```python
from build123d import *

# Parameters (mm, degrees)
BASE_FLANGE1_DEPTH = 20.1168
SKETCH6_R          = 2.4892
CUT_EXTRUDE1_DEPTH = 72.471393622
SKETCH7_R          = 5.08
CUT_EXTRUDE2_DEPTH = 71.156041481
FILLET1_R          = 3.175


# Read off the part's stored shape, not the designer's step: Base-Flange1
with BuildPart() as part:
    # Base-Flange1 outline → Base-Flange1 (new body)
    with BuildSketch(Plane(origin=(0, 0, 0), x_dir=(1, 0, 0), z_dir=(0, 1, 0))):
        with BuildLine():
            Line((3.429, 0), (63.5, 0))
            Line((63.5, 0), (63.5, 2.667))
            Line((63.5, 2.667), (3.429, 2.667))
            ThreePointArc((3.429, 2.667), (2.890184633, 2.890184633), (2.667, 3.429))
            Line((2.667, 3.429), (2.667, 28.575))
            Line((2.667, 28.575), (0, 28.575))
            Line((0, 28.575), (0, 3.429))
            ThreePointArc((0, 3.429), (1.004330847, 1.004330847), (3.429, 0))
        make_face()
    extrude(amount=BASE_FLANGE1_DEPTH)

    # Sketch6 → Cut-Extrude1 (cut, through all)
    with BuildSketch(Plane(origin=(0, 0, -2.667), x_dir=(-1, 0, 0), z_dir=(0, 0, -1))):
        with Locations((-50.8, 10.0584)):
            Circle(SKETCH6_R)
        with Locations((-38.1, 10.0584)):
            Circle(SKETCH6_R)
        with Locations((-25.4, 10.0584)):
            Circle(SKETCH6_R)
        with Locations((-12.7, 10.0584)):
            Circle(SKETCH6_R)
    extrude(amount=-CUT_EXTRUDE1_DEPTH, mode=Mode.SUBTRACT)

    # Sketch7 → Cut-Extrude2 (cut, through all)
    with BuildSketch(Plane(origin=(2.667, 0, 0), x_dir=(0, 0, -1), z_dir=(1, 0, 0))):
        with Locations((19.05, 10.0584)):
            Circle(SKETCH7_R)
    extrude(amount=-CUT_EXTRUDE2_DEPTH, mode=Mode.SUBTRACT)

    # Fillet1
    fillet1_edges = [part.edges().sort_by_distance(p)[0] for p in [
        (1.3335, 20.1168, -28.575),
        (1.3335, 0, -28.575),
        (63.5, 20.1168, -1.3335),
        (63.5, 0, -1.3335),
    ]]
    fillet(fillet1_edges, radius=FILLET1_R)


solid = part.part
```
For this review, take the finished solid that the model builds, in its own axes (mm). A direction names the side the tool comes from. Give positions to 0.01 mm unless a question says otherwise; leave off trailing zeros. Write each loop counter-clockwise with the first axis right and the second up, starting at its lowest first coordinate (ties: lowest second). Pieces come first, ordered by that corner, then holes.
Item 1: Wall thickness on probe 1 along Y at (x, z) = (38.1, -1.6); probe 2 along X at (y, z) = (13.75, -26); probe 3 along Z at (x, y) = (61.5, 18): over which ranges is each line inside the solid? List them lowest first.
Item 2: Take a section at A-A (y = 14.25). Give the boundary of the cut face in (x, z) (3 decimals), and give its area (3 significant figures).
Item 3: Machinability: for faces 5 (the face through (62.545, 19.211, -1.352)), 6 (the face through (34, 10, -2.667)), which of the approach directions +Z, -Z, +X, -X, +Y, -Y give a long, thin tool a straight path to every point of the face, cutting with its end or side? Answer none if there is none.
Item 4: Take a section at B-B (x = 25.4). Give the boundary of the cut face in (y, z).
Item 5: Take a section at C-C (z = -19.05). Give the boundary of the cut face in (x, y).
Item 6: Insertion check: P1, Ø10, axis at x = 45.5, y = 9, coming from the -Z side; P2, Ø6, axis at y = 10.06, z = -19.05, coming from the +X side; P3, Ø5.5, axis at x = 38.1, y = 10.06, coming from the +Z side; P4, Ø10, axis at y = 6, z = -14, coming from the +X side. Each pin has a flat end and moves straight along its axis. Give the tip position at first contact, or say it passes through.
Item 7: The part is to be moulded in two halves that separate along X. For faces 1 (the face through (0.98, 9.92, -1.03)), 2 (the face through (2.667, 10, -13)), 3 (the face through (23, 0, -2)), 4 (the face through (13.24, 7.63, -1.35)), say which applies: +X half, -X half, draft (parallel to the pull), parting line (faces both ways), or undercut.
Item 8: Take a section at D-D (y = 17.75). Give the boundary of the cut face in (x, z), and give its area (3 significant figures).
Established:
1. probe 1: y = 0 to 7.57, 12.55 to 20.12
1. probe 2: x = 0 to 2.67
1. probe 3: z = -2.67 to 0
2. outline: (0, -28.575) - (2.667, -28.575) - (2.667, -21.92) - (0, -21.92) - close; (0, -16.18) - (2.667, -16.18) - (2.667, -3.429) arc R0.762 cw to (3.429, -2.667) - (63.5, -2.667) - (63.5, 0) - (3.429, 0) arc R3.429 ccw to (0, -3.429) - close
2. area: 221 mm2
3. face 5: +Z, -Z, +X, +Y
3. face 6: -Z, +X, +Y, -Y
4. outline: (0, -2.67) - (7.57, -2.67) - (7.57, 0) - (0, 0) - close; (12.55, -2.67) - (20.12, -2.67) - (20.12, 0) - (12.55, 0) - close
5. outline: (0, 0) - (2.67, 0) - (2.67, 4.98) - (0, 4.98) - close; (0, 15.14) - (2.67, 15.14) - (2.67, 20.12) - (0, 20.12) - close
6. P1: stops at z = -2.67
6. P2: passes through
6. P3: stops at z = 0
6. P4: stops at x = 2.67
7. face 1: -X half
7. face 2: +X half
7. face 3: draft
7. face 4: undercut
8. outline: (0, -28.47) - (2.67, -28.47) - (2.67, -3.43) arc R0.76 cw to (3.43, -2.67) - (63.4, -2.67) - (63.4, 0) - (3.43, 0) arc R3.43 ccw to (0, -3.43) - close
8. area: 235 mm2
